Read the model definition and answer for the solid it produces. Units are mm, in the model's axes. A direction names the side the tool comes from. Give positions to 0.01 mm unless a question says otherwise; leave off trailing zeros. Write each loop counter-clockwise with the first axis right and the second up, starting at its lowest first coordinate (ties: lowest second). Pieces come first, ordered by that corner, then holes.
```python
from build123d import *

# Parameters (mm, degrees)
F0_W     = 17
F0_H     = 12
F1_DEPTH = 21
F2_DEPTH = 14


with BuildPart() as f1:
    # F0 (on Front) → F1 (new body)
    with BuildSketch(Plane.XZ):
        with Locations((1.5, 0)):
            Rectangle(F0_W, F0_H)
        Polygon((-5.196152, 0), (-2.598076, 4.5), (2.598076, 4.5), (5.196152, 0), (2.598076, -4.5), (-2.598076, -4.5), align=None, mode=Mode.SUBTRACT)
        Polygon((2.598076, 4.5), (-2.598076, 4.5), (-5.196152, 0), (-2.598076, -4.5), (2.598076, -4.5), (5.196152, 0), align=None)
    extrude(amount=F1_DEPTH)

    # F0 (on Front) → F2 (cut)
    with BuildSketch(Plane.XZ):
        Polygon((2.598076, 4.5), (-2.598076, 4.5), (-5.196152, 0), (-2.598076, -4.5), (2.598076, -4.5), (5.196152, 0), align=None)
    extrude(amount=F2_DEPTH, mode=Mode.SUBTRACT)


solid = f1.part
```
Item 1: Section B-B (x = -1.25) is taken. Write down the section's boundary in (y, z), and give its area (3 significant figures).
Result set:
outline: (-21, -6) - (0, -6) - (0, -4.5) - (-14, -4.5) - (-14, 4.5) - (0, 4.5) - (0, 6) - (-21, 6) - close
area: 126 mm2
Item 2: Section A-A (y = -9.75) is taken. Write down the section's boundary in (x, z), and give its area (3 significant figures).
Result set:
outline: (-7, -6) - (10, -6) - (10, 6) - (-7, 6) - close; hole (-5.2, 0) - (-2.6, -4.5) - (2.6, -4.5) - (5.2, 0) - (2.6, 4.5) - (-2.6, 4.5) - close
area: 134 mm2
Item 3: Which of the six approach directions +Z, -Z, +X, -X, +Y, -Y give full straight-line access (tool end or side, diameter ignored) to faces 1 (the flat face through (1, -10, 6)), 2 (the flat face through (0, -7, 4.5))?
Result set:
face 1: +Z, +X, -X, +Y, -Y
face 2: +Y
Item 4: This flat-tipped pin is pushed along its axis until it touches: pin 1 Ø2.5 at (x, z) = (-1.5, 0.5) entering from +Y. Where does it stop, or does it pass through?
Result set:
pin 1: stops at y = -14
Item 5: Determine the mould class of faces 3 (the flat face through (-7, -10, 0)), 4 (the flat face through (1, -10, -6)), 5 (the flat face through (-3.88, -6.9, 2.28)) for opening direction X: pulls with the +X half, pulls with the -X half, needs draft (parallel to the pull), parting line crosses it, or undercut.
Result set:
face 3: pulls with the -X half
face 4: needs draft
face 5: undercut
Item 6: Section C-C (z = 0.25) is taken. Write down the section's boundary in (x, y).
Result set:
outline: (-7, -21) - (10, -21) - (10, 0) - (5.05, 0) - (5.05, -14) - (-5.05, -14) - (-5.05, 0) - (-7, 0) - close
Item 7: Find the intervals of material crossed by line 1 along X through (y, z) = (-8, 1.5); line 2 along X through (y, z) = (-7.25, 0.25); line 3 along Y through (x, z) = (-2.5, 3.5), in increasing order.
Result set:
line 1: x = -7 to -4.33, 4.33 to 10
line 2: x = -7 to -5.05, 5.05 to 10
line 3: y = -21 to -14
